Autodesk Inventor part; units mm, degrees
ref_plane "YZ Plane" through (0, 0, 0) normal (1, 0, 0) x (0, 1, 0)
ref_plane "XZ Plane" through (0, 0, 0) normal (0, 1, 0) x (-1, 0, 0)
ref_plane "XY Plane" through (0, 0, 0) normal (0, 0, 1) x (1, 0, 0)
sketch "Sketch1" plane through (0, 0, 0) normal (0, 1, 0) x (-1, 0, 0)
  circle A0 centre (0, 0) radius 3.975
  circle A1 centre (0, 0) radius 1.6
  circle A2 centre (0, 0) radius 8
  dimension "d0" = 7.95
  dimension "d1" = 3.2
  dimension "d2" = 16
extrude "Extrusion1" add sketch "Sketch1" along normal blind 2 contours A0
extrude "Extrusion2" add sketch "Sketch1" against normal blind 3.8 contours A0 | A2
sketch "Sketch3" plane through (0, -3.8, 0) normal (0, -1, 0) x (1, 0, 0)
  line L0 (8, 0) -> (6, 0) construction
  line L1 (6, 0) -> (6, -6.7165)
  line L2 (6, 0) -> (6, 8)
  line L3 (6, 8) -> (11.3207, 8)
  line L4 (11.3207, 8) -> (13.7407, -4.0569)
  line L5 (13.7407, -4.0569) -> (10.7642, -6.413)
  line L6 (10.7642, -6.413) -> (6, -6.7165)
  dimension "d11" = 2
extrude "Extrusion4" cut sketch "Sketch3" against normal blind 6.75
mirror "Mirror1" about plane through (0, 0, 0) normal (1, 0, 0) of "Extrusion4"
sketch "Sketch4" plane through (0, -3.8, 0) normal (0, -1, 0) x (1, 0, 0)
  line L0 (-6, 5.2915) -> (-6, -5.2915)
  arc A0 (-6, -5.2915) -> (6, -5.2915) centre (0, 0) ccw
  line L1 (6, -5.2915) -> (6, 5.2915)
  arc A1 (6, 5.2915) -> (-6, 5.2915) centre (0, 0) ccw
  circle A2 centre (0, 0) radius 1.6
extrude "Extrusion5" cut sketch "Sketch4" against normal blind 1.75
properties part number "C-Channel Spacer M3"
Verification items for the finished model (mm, model axes). Coordinates: 2 decimals unless noted, no trailing zeros. Loops run counter-clockwise (first coordinate to the right, second up) from the corner with the lowest first, then second, coordinate; pieces in that order, holes last. Notation, with made-up numbers: (-14, 47.5) - (39, 47.5) arc R30 ccw to (39, 69.5) - close; hole circle Ø6 at (86, 44.5). An arc over 180 degrees is marked (long way). Answer as a JSON object with one key per item and string values.
(1) Mould release check, pull along X, two halves, no side actions. Record for faces 1 (the cylindrical face through (0.86, 0.99, 3.88)), 2 (the flat face through (4, 0, -2)), 3 (the cylindrical face through (1.27, -0.05, 0.97)): pulls with the +X half, pulls with the -X half, needs draft (parallel to the pull), parting line crosses it, or undercut.
Response:
{"face 1": "parting line crosses it", "face 2": "needs draft", "face 3": "undercut"}
(2) Cross-section at C-C, the plane y = -1.3. Record the boundary of the cut face in (x, z), then the cut area to 3 significant figures.
Response:
{"outline": "(-6, -5.29) arc R8 ccw to (6, -5.29) - (6, 5.29) arc R8 ccw to (-6, 5.29) - close; hole circle Ø3.2 at (0, 0)", "area": "164 mm²"}
(3) Cross-section at B-B, the plane z = 0. Record the boundary of the cut face in (x, y) (3 decimals), then the cut area to 3 significant figures.
Response:
{"outline": "(-6, -2.05) - (-1.6, -2.05) - (-1.6, 2) - (-3.975, 2) - (-3.975, 0) - (-6, 0) - close; (1.6, -2.05) - (6, -2.05) - (6, 0) - (3.975, 0) - (3.975, 2) - (1.6, 2) - close", "area": "27.5 mm²"}
(4) Scan lines: line 1 along Z through (x, y) = (0, 1.15) (3 decimals); line 2 along X through (y, z) = (-1.15, 0); line 3 along X through (y, z) = (-1.4, -1). Record each from-to range of solid material in increasing order.
Response:
{"line 1": "z = -3.975 to -1.6, 1.6 to 3.975", "line 2": "x = -6 to -1.6, 1.6 to 6", "line 3": "x = -6 to -1.25, 1.25 to 6"}
(5) Cross-section at A-A, the plane x = 0. Record the boundary of the cut face in (y, z) (3 decimals).
Response:
{"outline": "(-2.05, -8) - (0, -8) - (0, -3.975) - (2, -3.975) - (2, -1.6) - (-2.05, -1.6) - close; (-2.05, 1.6) - (2, 1.6) - (2, 3.975) - (0, 3.975) - (0, 8) - (-2.05, 8) - close"}
(6) Cross-section at D-D, the plane z = -2.75. Record the boundary of the cut face in (x, y).
Response:
{"outline": "(-6, -2.05) - (6, -2.05) - (6, 0) - (2.87, 0) - (2.87, 2) - (-2.87, 2) - (-2.87, 0) - (-6, 0) - close"}
